Read the model definition and answer for the solid it produces. Units are mm, in the model's axes. Coordinates: 2 decimals unless noted, no trailing zeros. Loops run counter-clockwise (first coordinate to the right, second up) from the corner with the lowest first, then second, coordinate; pieces in that order, holes last. Notation, with made-up numbers: (-33, -15) - (23, -15) arc R14 ccw to (23, 8) - close; hole circle Ø7 at (82.5, 89.5). An arc over 180 degrees is marked (long way). Use one line per item in the form item = value.
from build123d import *

# Parameters (mm, degrees)
F1_DEPTH = 6
F3_DEPTH = 3


with BuildPart() as f1:
    # F0 (on Top) → F1 (new body)
    with BuildSketch(Plane.XY):
        with BuildLine():
            Line((84.748961, 75.975446), (-25.751039, 75.975446))
            ThreePointArc((-25.751039, 75.975446), (-29.286573, 74.51098), (-30.751039, 70.975446))
            Line((-30.751039, 70.975446), (-30.751039, 8.284529))
            ThreePointArc((-30.751039, 8.284529), (-34.728897, -5.362881), (-45.416535, -14.735688))
            Line((-45.416535, -14.735688), (-109.711543, -44.716943))
            ThreePointArc((-109.711543, -44.716943), (-112.660436, -47.539893), (-113.281446, -51.574663))
            Line((-113.281446, -51.574663), (-106.642219, -89.227591))
            ThreePointArc((-106.642219, -89.227591), (-104.586062, -92.45511), (-100.849939, -93.283389))
            Line((-100.849939, -93.283389), (86.138146, -60.312344))
            ThreePointArc((86.138146, -60.312344), (90.877316, -57.576183), (92.748961, -52.433882))
            Line((92.748961, -52.433882), (92.748961, 67.975446))
            ThreePointArc((92.748961, 67.975446), (90.405815, 73.632301), (84.748961, 75.975446))
        make_face()
        with BuildLine():
            Line((-21.694494, -38.430323), (-90.755147, -70.633835))
            ThreePointArc((-90.755147, -70.633835), (-94.077462, -69.424611), (-92.868238, -66.102296))
            Line((-92.868238, -66.102296), (-23.807585, -33.898784))
            ThreePointArc((-23.807585, -33.898784), (-20.48527, -35.108008), (-21.694494, -38.430323))
        make_face(mode=Mode.SUBTRACT)
        with BuildLine():
            Line((51.23412, -60.882019), (-98.850581, -87.346002))
            ThreePointArc((-98.850581, -87.346002), (-101.746721, -85.318103), (-99.718822, -82.421963))
            Line((-99.718822, -82.421963), (50.36588, -55.957981))
            ThreePointArc((50.36588, -55.957981), (53.262019, -57.98588), (51.23412, -60.882019))
        make_face(mode=Mode.SUBTRACT)
        with BuildLine():
            Line((-34.394494, -21.181494), (-103.455147, -53.385005))
            ThreePointArc((-103.455147, -53.385005), (-106.777462, -52.175782), (-105.568238, -48.853467))
            Line((-105.568238, -48.853467), (-36.507585, -16.649955))
            ThreePointArc((-36.507585, -16.649955), (-33.18527, -17.859179), (-34.394494, -21.181494))
        make_face(mode=Mode.SUBTRACT)
        with BuildLine():
            Line((-25.251039, -20.924554), (-25.251039, 67.975446))
            ThreePointArc((-25.251039, 67.975446), (-22.751039, 70.475446), (-20.251039, 67.975446))
            Line((-20.251039, 67.975446), (-20.251039, -20.924554))
            ThreePointArc((-20.251039, -20.924554), (-22.751039, -23.424554), (-25.251039, -20.924554))
        make_face(mode=Mode.SUBTRACT)
        with BuildLine():
            Line((-4.251039, -46.324554), (-4.251039, 67.975446))
            ThreePointArc((-4.251039, 67.975446), (-1.751039, 70.475446), (0.748961, 67.975446))
            Line((0.748961, 67.975446), (0.748961, -46.324554))
            ThreePointArc((0.748961, -46.324554), (-1.751039, -48.824554), (-4.251039, -46.324554))
        make_face(mode=Mode.SUBTRACT)
        with BuildLine():
            Line((16.748961, -46.324554), (16.748961, 67.975446))
            ThreePointArc((16.748961, 67.975446), (19.248961, 70.475446), (21.748961, 67.975446))
            Line((21.748961, 67.975446), (21.748961, -46.324554))
            ThreePointArc((21.748961, -46.324554), (19.248961, -48.824554), (16.748961, -46.324554))
        make_face(mode=Mode.SUBTRACT)
        with BuildLine():
            Line((37.748961, -46.324554), (37.748961, 67.975446))
            ThreePointArc((37.748961, 67.975446), (40.248961, 70.475446), (42.748961, 67.975446))
            Line((42.748961, 67.975446), (42.748961, -46.324554))
            ThreePointArc((42.748961, -46.324554), (40.248961, -48.824554), (37.748961, -46.324554))
        make_face(mode=Mode.SUBTRACT)
        with BuildLine():
            Line((58.748961, -46.324554), (58.748961, 67.975446))
            ThreePointArc((58.748961, 67.975446), (61.248961, 70.475446), (63.748961, 67.975446))
            Line((63.748961, 67.975446), (63.748961, -46.324554))
            ThreePointArc((63.748961, -46.324554), (61.248961, -48.824554), (58.748961, -46.324554))
        make_face(mode=Mode.SUBTRACT)
        with BuildLine():
            Line((79.748961, -46.324554), (79.748961, 67.975446))
            ThreePointArc((79.748961, 67.975446), (82.248961, 70.475446), (84.748961, 67.975446))
            Line((84.748961, 67.975446), (84.748961, -46.324554))
            ThreePointArc((84.748961, -46.324554), (82.248961, -48.824554), (79.748961, -46.324554))
        make_face(mode=Mode.SUBTRACT)
    extrude(amount=F1_DEPTH)

    # F2 (on face) → F3 (cut)
    with BuildSketch(Plane(origin=(0, 0, 0), x_dir=(1, 0, 0), z_dir=(0, 0, -1))):
        with BuildLine():
            ThreePointArc((87.248961, 46.324554), (82.248961, 51.324554), (77.248961, 46.324554))
            Line((77.248961, 46.324554), (77.248961, -67.975446))
            ThreePointArc((77.248961, -67.975446), (82.248961, -72.975446), (87.248961, -67.975446))
            Line((87.248961, -67.975446), (87.248961, 46.324554))
        make_face()
        with BuildLine():
            ThreePointArc((66.248961, 46.324554), (61.248961, 51.324554), (56.248961, 46.324554))
            Line((56.248961, 46.324554), (56.248961, -67.975446))
            ThreePointArc((56.248961, -67.975446), (61.248961, -72.975446), (66.248961, -67.975446))
            Line((66.248961, -67.975446), (66.248961, 46.324554))
        make_face()
        with BuildLine():
            ThreePointArc((45.248961, 46.324554), (40.248961, 51.324554), (35.248961, 46.324554))
            Line((35.248961, 46.324554), (35.248961, -67.975446))
            ThreePointArc((35.248961, -67.975446), (40.248961, -72.975446), (45.248961, -67.975446))
            Line((45.248961, -67.975446), (45.248961, 46.324554))
        make_face()
        with BuildLine():
            ThreePointArc((24.248961, 46.324554), (19.248961, 51.324554), (14.248961, 46.324554))
            Line((14.248961, 46.324554), (14.248961, -67.975446))
            ThreePointArc((14.248961, -67.975446), (19.248961, -72.975446), (24.248961, -67.975446))
            Line((24.248961, -67.975446), (24.248961, 46.324554))
        make_face()
        with BuildLine():
            ThreePointArc((3.248961, 46.324554), (-1.751039, 51.324554), (-6.751039, 46.324554))
            Line((-6.751039, 46.324554), (-6.751039, -67.975446))
            ThreePointArc((-6.751039, -67.975446), (-1.751039, -72.975446), (3.248961, -67.975446))
            Line((3.248961, -67.975446), (3.248961, 46.324554))
        make_face()
        with BuildLine():
            ThreePointArc((-24.864131, 31.633015), (-18.2195, 34.051462), (-20.637948, 40.696092))
            Line((-20.637948, 40.696092), (-89.698601, 72.899604))
            ThreePointArc((-89.698601, 72.899604), (-96.343232, 70.481156), (-93.924784, 63.836526))
            Line((-93.924784, 63.836526), (-24.864131, 31.633015))
        make_face()
        with BuildLine():
            ThreePointArc((-17.751039, 20.924554), (-22.751039, 25.924554), (-27.751039, 20.924554))
            Line((-27.751039, 20.924554), (-27.751039, -67.975446))
            ThreePointArc((-27.751039, -67.975446), (-22.751039, -72.975446), (-17.751039, -67.975446))
            Line((-17.751039, -67.975446), (-17.751039, 20.924554))
        make_face()
        with BuildLine():
            ThreePointArc((-37.564131, 14.384186), (-30.9195, 16.802633), (-33.337948, 23.447263))
            Line((-33.337948, 23.447263), (-102.398601, 55.650775))
            ThreePointArc((-102.398601, 55.650775), (-109.043232, 53.232327), (-106.624784, 46.587697))
            Line((-106.624784, 46.587697), (-37.564131, 14.384186))
        make_face()
        with BuildLine():
            ThreePointArc((49.931759, 53.495961), (55.724039, 57.551759), (51.668241, 63.344039))
            Line((51.668241, 63.344039), (-98.416461, 89.808021))
            ThreePointArc((-98.416461, 89.808021), (-104.20874, 85.752223), (-100.152942, 79.959944))
            Line((-100.152942, 79.959944), (49.931759, 53.495961))
        make_face()
    extrude(amount=-F3_DEPTH, mode=Mode.SUBTRACT)


solid = f1.part
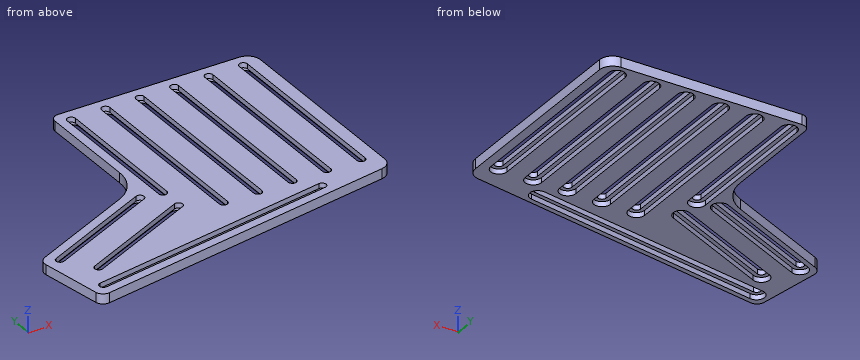
Item 1: Each of these flat-tipped pins is pushed along its axis until it touches: P1, Ø1, axis at x = -17.5, z = 3, coming from the -Y side; P2, Ø3, axis at x = -71, z = 4.5, coming from the +Y side; P3, Ø3, axis at y = 30.5, z = 1.5, coming from the -X side. Where does it stop, or does it pass through?
Results below:
P1 = -78.67
P2 = -25.97
P3 = -30.75
Item 2: The part is cut by section B-B on z = 2. Count the separate pieces of the cut face and the enclosed holes in it, plus the area to 3 significant figures.
Results below:
separate_pieces = 1
enclosed_holes = 9
area = 12,600 mm²
Item 3: The part is cut by section A-A on x = -60.5. Give the vertices of the cut face in (y, z).
Results below:
outline = (-86.17, 0) - (-83.12, 0) - (-83.12, 3) - (-80.58, 3) - (-80.58, 6) - (-86.17, 6) - close; (-75.51, 3) - (-72.97, 3) - (-72.97, 0) - (-59.28, 0) - (-59.28, 3) - (-56.53, 3) - (-56.53, 6) - (-75.51, 6) - close; (-51.01, 3) - (-48.25, 3) - (-48.25, 0) - (-36.11, 0) - (-36.11, 3) - (-33.35, 3) - (-33.35, 6) - (-51.01, 6) - close; (-27.84, 3) - (-25.08, 3) - (-25.08, 0) - (-21.77, 0) - (-21.77, 6) - (-27.84, 6) - close
Item 4: Find the intervals of material crossed by L1, parallel to Y at x = 40, z = 4.15; L2, parallel to Y at x = -50, z = 1.5; L3, parallel to Y at x = -53.5, z = 4.45, in increasing order.
Results below:
L1 = -68.45 to -62.86, -57.79 to -48.81, 70.46 to 75.98
L2 = -84.32 to -81.27, -71.12 to -54.39, -43.35 to -31.22, -20.18 to -16.87
L3 = -84.93 to -79.35, -74.27 to -53.26, -47.74 to -30.09, -24.57 to -18.51
Item 5: The part is cut by section C-C on x = -14. Give the vertices of the cut face in (y, z), plus the area to 3 significant figures.
Results below:
outline = (-77.97, 0) - (-74.92, 0) - (-74.92, 3) - (-72.38, 3) - (-72.38, 6) - (-77.97, 6) - close; (-67.31, 3) - (-64.77, 3) - (-64.77, 0) - (75.98, 0) - (75.98, 6) - (-67.31, 6) - close
area = 878 mm²
